For this review, take the finished solid that the model builds, in its own axes (mm). A direction names the side the tool comes from. Give positions to 0.01 mm unless a question says otherwise; leave off trailing zeros. Loops run counter-clockwise (first coordinate to the right, second up) from the corner with the lowest first, then second, coordinate; pieces in that order, holes last. Notation, with made-up numbers: (-2.75, 7.25) -> (16.25, 7.25) arc R32 ccw to (16.25, 41.25) -> close; hole circle Ø7 at (82.25, 57.25). An arc over 180 degrees is marked (long way). Answer as CSV lines item,"result". Start each with the question number.
Item 1: Machinability: for faces 4 (the face through (2.6, -6.35, 0.1)), 5 (the face through (-2.14, -3.13, -2.1)), which of the approach directions +Z, -Z, +X, -X, +Y, -Y give a long, thin tool a straight path to every point of the face, cutting with its end or side? Answer none if there is none.
Item 2: Add section A-A on y = -1.75. State the section outline as (x, z) points, plus the area to 3 significant figures.
Item 3: For L1, parallel to Z at x = -0.5, y = -2.75; L2, parallel to X at y = -6, z = -1; L3, parallel to X at y = -3.5, z = -0.75, list the stretches that pass through material, from the lowest coordinate up. Write a range as from..to.
Item 4: Add section D-D on x = 4.25. State the section outline as (y, z) points, plus the area to 3 significant figures.
Item 5: Add section C-C on z = 0.5. State the section outline as (x, y) points.
Item 6: The part is to be moulded in two halves that separate along X. For faces 1 (the face through (2.14, -3.13, 2.1)), 2 (the face through (2.6, 0, 0.1)), 3 (the face through (-6, -3, 0)), say which applies: +X half, -X half, draft (parallel to the pull), parting line (faces both ways), or undercut.
Item 7: Add section B-B on x = 0.75. State the section outline as (y, z) points.
Item 8: Clearance check with flat-ended pins moving along their axes: P1, Ø0.8, axis at y = -4, z = -4, coming from the -X side; P2, Ø2, axis at y = -3, z = -4, coming from the +X side; P3, Ø0.8, axis at x = -4, y = -1.5, coming from the -Z side. State where each tip first meets the part, or that it passes through.
```python
from build123d import *

# Parameters (mm, degrees)
F0_R     = 6
F0_R_2   = 2
F1_DEPTH = 6.35


# Not quite as in the source:
# - a length typed as a fraction of an inch, garbled in the dataset ("3 / 203.2 mm" for 3/8 in), is restored


with BuildPart() as f1:
    # F0 (on Front) → F1 (new body)
    with BuildSketch(Plane.XZ):
        Circle(F0_R)
        with BuildLine():
            ThreePointArc((0, 4.5), (3.1819805153, 3.1819805153), (4.5, 0))
            ThreePointArc((4.5, 0), (3.1819805153, -3.1819805153), (0, -4.5))
            ThreePointArc((0, -4.5), (-3.1819805153, -3.1819805153), (-4.5, 0))
            ThreePointArc((-4.5, 0), (-3.1819805153, 3.1819805153), (0, 4.5))
        make_face(mode=Mode.SUBTRACT)
        with BuildLine():
            ThreePointArc((0, -4.5), (3.1819805153, -3.1819805153), (4.5, 0))
            Line((4.5, 0), (3, 0))
            ThreePointArc((3, 0), (2.1213203436, -2.1213203436), (0, -3))
            Line((0, -3), (0, -4.5))
        make_face()
        with BuildLine():
            ThreePointArc((0, -3), (2.1213203436, -2.1213203436), (3, 0))
            ThreePointArc((3, 0), (2.1213203436, 2.1213203436), (0, 3))
            ThreePointArc((0, 3), (-2.1213203436, 2.1213203436), (-3, 0))
            ThreePointArc((-3, 0), (-2.1213203436, -2.1213203436), (0, -3))
        make_face()
        Circle(F0_R_2, mode=Mode.SUBTRACT)
        with BuildLine():
            Line((0, 3), (0, 4.5))
            ThreePointArc((0, 4.5), (-3.1819805153, 3.1819805153), (-4.5, 0))
            Line((-4.5, 0), (-3, 0))
            ThreePointArc((-3, 0), (-2.1213203436, 2.1213203436), (0, 3))
        make_face()
    extrude(amount=F1_DEPTH)


solid = f1.part
```
Computed values:
1,face 4,"+Z, -Z, +X, -X, -Y"
1,face 5,"+Y, -Y"
2,outline,"circle Ø12 at (0, 0); hole (-4.5, 0) arc R4.5 ccw to (0, -4.5) -> (0, -3) arc R3 cw to (-3, 0) -> close; hole circle Ø4 at (0, 0); hole (0, 3) arc R3 cw to (3, 0) -> (4.5, 0) arc R4.5 ccw to (0, 4.5) -> close"
2,area,"82.9 mm²"
3,L1,"-5.98..-4.47, -2.96..-1.94, 1.94..5.98"
3,L2,"-5.92..-4.39, -2.83..-1.73, 1.73..5.92"
3,L3,"-5.95..-4.44, -2.9..-1.85, 1.85..5.95"
4,outline,"(-6.35, -4.24) -> (0, -4.24) -> (0, 0) -> (-6.35, 0) -> close; (-6.35, 1.48) -> (0, 1.48) -> (0, 4.24) -> (-6.35, 4.24) -> close"
4,area,"44.4 mm²"
5,outline,"(-5.98, -6.35) -> (-1.94, -6.35) -> (-1.94, 0) -> (-5.98, 0) -> close; (1.94, -6.35) -> (2.96, -6.35) -> (2.96, 0) -> (1.94, 0) -> close; (4.47, -6.35) -> (5.98, -6.35) -> (5.98, 0) -> (4.47, 0) -> close"
6,face 1,"undercut"
6,face 2,"draft"
6,face 3,"parting line"
7,outline,"(-6.35, -5.95) -> (0, -5.95) -> (0, -1.85) -> (-6.35, -1.85) -> close; (-6.35, 1.85) -> (0, 1.85) -> (0, 2.9) -> (-6.35, 2.9) -> close; (-6.35, 4.44) -> (0, 4.44) -> (0, 5.95) -> (-6.35, 5.95) -> close"
8,P1,"x = -4.8"
8,P2,"x = 5.2"
8,P3,"z = -4.8"
